The model under review builds one solid part; all positions refer to its coordinate system, in mm. A direction names the side the tool comes from. Coordinates: 2 decimals unless noted, no trailing zeros. Loops run counter-clockwise (first coordinate to the right, second up) from the corner with the lowest first, then second, coordinate; pieces in that order, holes last. Notation, with made-up numbers: M 49,1.5 L 74,1.5 A23 ccw 74,14.5 Z; hole C 22.5,38 d10. An arc over 180 degrees is marked long. Write item = value, one per line. Start each with the question number.
Q1. We need section A-A on x = 24. Give the boundary of the cut face in (y, z).
Q2. Clearance check with flat-ended pins moving along their axes: pin 1 Ø7 at (x, z) = (27, 4.5) entering from +Y; pin 2 Ø0.9 at (x, y) = (-27.5, 1) entering from -Z; pin 3 Ø5.5 at (y, z) = (10, 1) entering from -X. State where each tip first meets the part, or that it passes through.
Q3. We need section D-D on z = 3. Give the boundary of the cut face in (x, y), and give its area (3 significant figures).
Q4. For faces 1 (the face through (28, 1, 1.75)), 2 (the face through (-28, 1, -1.75)), 3 (the face through (-27, 3, 3)), 4 (the face through (26, 3, -3)), list the 3-axis set-ups (+Z, -Z, +X, -X, +Y, -Y) from which the entire face can be reached by the end or side of a thin tool; tool diameter is ignored.
Q5. We need section C-C on y = 8.5. Give the boundary of the cut face in (x, z), and give its area (3 significant figures).
Q6. Wall thickness on probe 1 along X at (y, z) = (16.5, 9); probe 2 along Z at (x, y) = (29, 2.75): over which ranges is each line inside the solid? List them lowest first.
Q7. We need section B-B on z = -8. Give the boundary of the cut face in (x, y), and give its area (3 significant figures).
from build123d import *

# Parameters (mm, degrees)
SKETCH1_W           = 46
SKETCH1_H           = 32
BOSS_EXTRUDE1_DEPTH = 18
BOSS_EXTRUDE2_DEPTH = 3


with BuildPart() as part:
    # Sketch1 → Boss-Extrude1 (new body)
    with BuildSketch(Plane(origin=(0, 0, 0), x_dir=(1, 0, 0), z_dir=(0, 1, 0))):
        Rectangle(SKETCH1_W, SKETCH1_H)
    extrude(amount=BOSS_EXTRUDE1_DEPTH)

    # Sketch2 → Boss-Extrude2 (add)
    with BuildSketch(Plane(origin=(0, 0, 0), x_dir=(1, 0, 0), z_dir=(0, 1, 0))):
        with BuildLine():
            Line((-31, 1.75), (-24.75, 1.75))
            ThreePointArc((-24.75, 1.75), (-23.512563133, 1.237436867), (-23, 0))
            Line((-23, 0), (-23, 6.5))
            Line((-23, 6.5), (-31.319224576, 3.697679096))
            ThreePointArc((-31.319224576, 3.697679096), (-31.98683309, 2.58825807), (-31, 1.75))
        make_face()
        with BuildLine():
            Line((-23, -6.5), (-23, 0))
            ThreePointArc((-23, 0), (-23.512563133, -1.237436867), (-24.75, -1.75))
            Line((-24.75, -1.75), (-31, -1.75))
            ThreePointArc((-31, -1.75), (-31.98683309, -2.58825807), (-31.319224576, -3.697679096))
            Line((-31.319224576, -3.697679096), (-23, -6.5))
        make_face()
        with BuildLine():
            Line((31.319224576, 3.697679096), (23, 6.5))
            Line((23, 6.5), (23, 0))
            ThreePointArc((23, 0), (23.512563133, 1.237436867), (24.75, 1.75))
            Line((24.75, 1.75), (31, 1.75))
            ThreePointArc((31, 1.75), (31.98683309, 2.58825807), (31.319224576, 3.697679096))
        make_face()
        with BuildLine():
            ThreePointArc((24.75, -1.75), (23.512563133, -1.237436867), (23, 0))
            Line((23, 0), (23, -6.5))
            Line((23, -6.5), (31.319224576, -3.697679096))
            ThreePointArc((31.319224576, -3.697679096), (31.98683309, -2.58825807), (31, -1.75))
            Line((31, -1.75), (24.75, -1.75))
        make_face()
    extrude(amount=BOSS_EXTRUDE2_DEPTH)


solid = part.part
Returned:
q1.outline = M 0,-6.16 L 3,-6.16 L 3,-1.58 L 0,-1.58 Z; M 0,1.58 L 3,1.58 L 3,6.16 L 0,6.16 Z
q2.pin_1 = 3
q2.pin_2 = -5.14
q2.pin_3 = -23
q3.outline = M -31.97,0 L 31.97,0 L 31.97,3 L 23,3 L 23,18 L -23,18 L -23,3 L -31.97,3 Z
q3.area = 882 mm^2
q4.face_1 = +X, +Y, -Y
q4.face_2 = -X, +Y, -Y
q4.face_3 = +Z, -Z, -X, +Y
q4.face_4 = +Z, -Z, +X, +Y
q5.outline = M -23,-16 L 23,-16 L 23,16 L -23,16 Z
q5.area = 1,470 mm^2
q6.probe_1 = -23 to 23
q6.probe_2 = -4.48 to -1.75, 1.75 to 4.48
q7.outline = M -23,0 L 23,0 L 23,18 L -23,18 Z
q7.area = 828 mm^2
